CAD build for the part. Positions are in the model's coordinates, mm. Round coordinates to 2 decimals unless told otherwise and drop trailing zeros. Write each loop counter-clockwise with the first axis right and the second up, starting at its lowest first coordinate (ties: lowest second). Pieces come first, ordered by that corner, then holes. Notation, with made-up numbers: (35.5, 8.5) -> (63.5, 8.5) arc R21 ccw to (63.5, 47.5) -> close; hole circle Ø6 at (-18, -34). An arc over 180 degrees is marked (long way). Put each result on its own line as item: value. Start each with the question number.
1. Flat gauge pins, fed straight in: P1, Ø4, axis at x = -4.5, z = 2.5, coming from the +Y side; P2, Ø2, axis at x = -6.6, z = 5.03, coming from the +Y side. Where does each tip first touch, or does it go through?
2. Saw through at A-A on x = 0. List the corners of the cut face in (y, z) (3 decimals).
3. Saw through at C-C on y = -0.8. List the corners of the cut face in (x, z) (3 decimals).
4. Saw through at B-B on z = 0. List the corners of the cut face in (x, y) (3 decimals), and give its area (3 significant figures).
5. Saw through at D-D on z = 6. List the corners of the cut face in (x, y) (3 decimals), and give its area (3 significant figures).
6. Drill centre lines: line 1 (Z direction, x = -6.5, y = -0.15); line 2 (Z direction, x = 0, y = -2.15); line 3 (Z direction, x = 5.25, y = -1.1). Where is each one in solid material? Low to high. Write a range as from..to.
7. Pull direction Z, two halves, no side cores. Call faces 1 (the cylindrical face through (-7.401, -1.565, 3.497)), 2 (the flat face through (0, -2, 7.95)), 3 (the cylindrical face through (-0.86, -1.57, -3.88)), 4 (the flat face through (-9.525, -2, 0)): pulls with the +Z half, pulls with the -Z half, needs draft (parallel to the pull), parting line crosses it, or undercut.
from build123d import *

# Parameters (mm, degrees)
F0_W     = 19.05
F0_H     = 15.5702
F0_R     = 3.9751
F1_DEPTH = 3.175
F3_D     = 3.4544


with BuildPart() as f1:
    # F0 (on Front) → F1 (new body)
    with BuildSketch(Plane.XZ):
        with Locations((0, 0.1651)):
            Rectangle(F0_W, F0_H)
        Circle(F0_R, mode=Mode.SUBTRACT)
    extrude(amount=F1_DEPTH)

    # F3 (through all)
    with Locations(Plane.XZ.offset(3.175)):
        with Locations((-6.604, 5.0292), (6.604, 5.0292), (6.604, -4.318), (-6.604, -4.318)):
            Hole(F3_D / 2)


solid = f1.part
Return value:
1. P1: stops at y = 0
1. P2: passes through
2. outline: (-3.175, -7.62) -> (0, -7.62) -> (0, -3.975) -> (-3.175, -3.975) -> close; (-3.175, 3.975) -> (0, 3.975) -> (0, 7.95) -> (-3.175, 7.95) -> close
3. outline: (-9.525, -7.62) -> (9.525, -7.62) -> (9.525, 7.95) -> (-9.525, 7.95) -> close; hole circle Ø3.454 at (-6.604, -4.318); hole circle Ø3.454 at (-6.604, 5.029); hole circle Ø7.95 at (0, 0); hole circle Ø3.454 at (6.604, -4.318); hole circle Ø3.454 at (6.604, 5.029)
4. outline: (-9.525, -3.175) -> (-3.975, -3.175) -> (-3.975, 0) -> (-9.525, 0) -> close; (3.975, -3.175) -> (9.525, -3.175) -> (9.525, 0) -> (3.975, 0) -> close
4. area: 35.2 mm^2
5. outline: (-9.525, -3.175) -> (-8.033, -3.175) -> (-8.033, 0) -> (-9.525, 0) -> close; (-5.175, -3.175) -> (5.175, -3.175) -> (5.175, 0) -> (-5.175, 0) -> close; (8.033, -3.175) -> (9.525, -3.175) -> (9.525, 0) -> (8.033, 0) -> close
5. area: 42.3 mm^2
6. line 1: z = -7.62..-6.04, -2.59..3.31, 6.75..7.95
6. line 2: z = -7.62..-3.98, 3.98..7.95
6. line 3: z = -7.62..-5.39, -3.25..3.96, 6.1..7.95
7. face 1: undercut
7. face 2: pulls with the +Z half
7. face 3: undercut
7. face 4: needs draft
